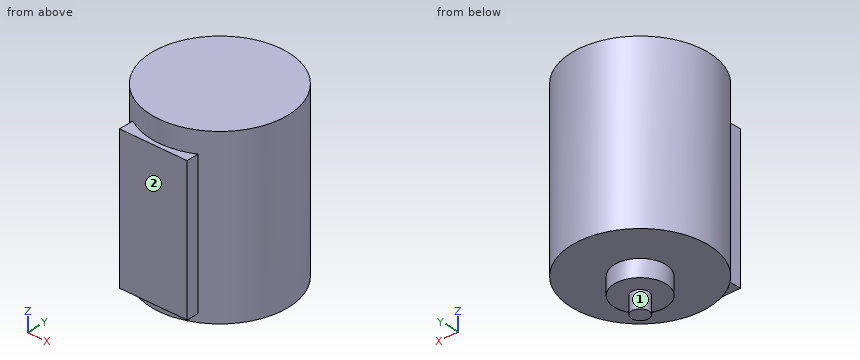
Solid Edge part; units mm, degrees
sketch "Sketch1" plane through (0, 0, 0) normal (0, 0, 1) x (1, 0, 0)
  circle A0 centre (-48.678, 43.9628) radius 40
extrude "Protrusion1" add sketch "Sketch1" along normal blind 100
sketch "Sketch2" plane through (0, 0, 0) normal (0, 0, 1) x (1, 0, 0)
  circle A0 centre (-48.678, 43.9628) radius 15
extrude "ExtrudedProtrusion_3" add sketch "Sketch2" against normal blind 10
sketch "Sketch3" plane through (-48.678, 43.9628, -10) normal (0, 0, -1) x (0, -1, 0)
  circle A0 centre (0, 0) radius 5
extrude "ExtrudedProtrusion_4" add sketch "Sketch3" along normal blind 10
sketch "Sketch4" plane through (-30, 0, 0) normal (1, 0, 0) x (0, 1, 0)
  line L0 (1.3522, 87.4748) -> (1.3522, 4.6806)
  line L1 (1.3522, 4.6806) -> (9.8812, 4.6806)
  line L2 (9.8812, 4.6806) -> (9.8812, 87.4748)
  line L3 (9.8812, 87.4748) -> (1.3522, 87.4748)
extrude "ExtrudedProtrusion_6" add sketch "Sketch4" against normal blind 40
Can you work these out from the model? Positions are in its coordinate system, mm. Face numbers are marked on the shaded views. A direction names the side the tool comes from. Coordinates: 2 decimals unless noted, no trailing zeros. Loops run counter-clockwise (first coordinate to the right, second up) from the corner with the lowest first, then second, coordinate; pieces in that order, holes last.
Item 1: Suppose I cut it at A-A (z = 38.5). Please give me the cut outline in (x, y).
Answers below:
outline: (-70, 1.35) - (-30, 1.35) - (-30, 8.59) arc R40 ccw (long way) to (-69.62, 9.88) - (-70, 9.88) - close
Item 2: Suppose I cut it at B-B (y = 35). Please give me the cut outline in (x, z).
Answers below:
outline: (-87.66, 0) - (-60.71, 0) - (-60.71, -10) - (-36.65, -10) - (-36.65, 0) - (-9.7, 0) - (-9.7, 100) - (-87.66, 100) - close
Item 3: Suppose I cut it at C-C (x = -55.5). Please give me the cut outline in (y, z), then the cut area to 3 significant figures.
Answers below:
outline: (1.35, 4.68) - (4.55, 4.68) - (4.55, 0) - (30.6, 0) - (30.6, -10) - (57.32, -10) - (57.32, 0) - (83.38, 0) - (83.38, 100) - (4.55, 100) - (4.55, 87.47) - (1.35, 87.47) - close
area: 8,410 mm2
Item 4: Which directions (+Z, -Z, +X, -X, +Y, -Y) give clear straight access to the entire face, cutting with the end or side of a thin tool? Please do the marked faces 1 and 2.
Answers below:
face 1: -Z
face 2: +Z, -Z, +X, -X, -Y
Item 5: Please list where these lines run through material, in increasing order: L1, parallel to Z at x = -32, y = 57; L2, parallel to Z at x = -45, y = 37; L3, parallel to Y at x = -38, z = 21.5.
Answers below:
L1: z = 0 to 100
L2: z = -10 to 100
L3: y = 1.35 to 82.51
Item 6: I'm going to push flat-ended pins straight in: pin 1 (7 mm diameter, centred on x = -55.5, y = 6, fed in from -Z); pin 2 (5 mm diameter, centred on y = 53.5, z = 44.5, fed in from +X); pin 3 (3 mm diameter, centred on x = -78, z = 15, fed in from +Y); pin 4 (10 mm diameter, centred on x = -73, z = 61, fed in from -Y). Where does each tip first touch, or does it pass through?
Answers below:
pin 1: stops at z = 0
pin 2: stops at x = -9.3
pin 3: stops at y = 72.7
pin 4: stops at y = 1.35
Item 7: Suppose I cut it at D-D (x = -25). Please give me the cut outline in (y, z), then the cut area to 3 significant figures.
Answers below:
outline: (11.72, 0) - (76.2, 0) - (76.2, 100) - (11.72, 100) - close
area: 6,450 mm2
